The drawing under review shows one solid part. Ordinate dimensions are in mm from its lowest x, y, z. A direction names the side the tool comes from. Coordinates: 2 decimals unless noted, no trailing zeros. Loops run counter-clockwise (first coordinate to the right, second up) from the corner with the lowest first, then second, coordinate; pieces in that order, holes last. Notation, with made-up numbers: (-15, -1) -> (3, -1) arc R13 ccw to (3, 5) -> close; hole circle Ø3 at (64, -33). An arc over 180 degrees is marked (long way). Use a Markdown table: item, result.
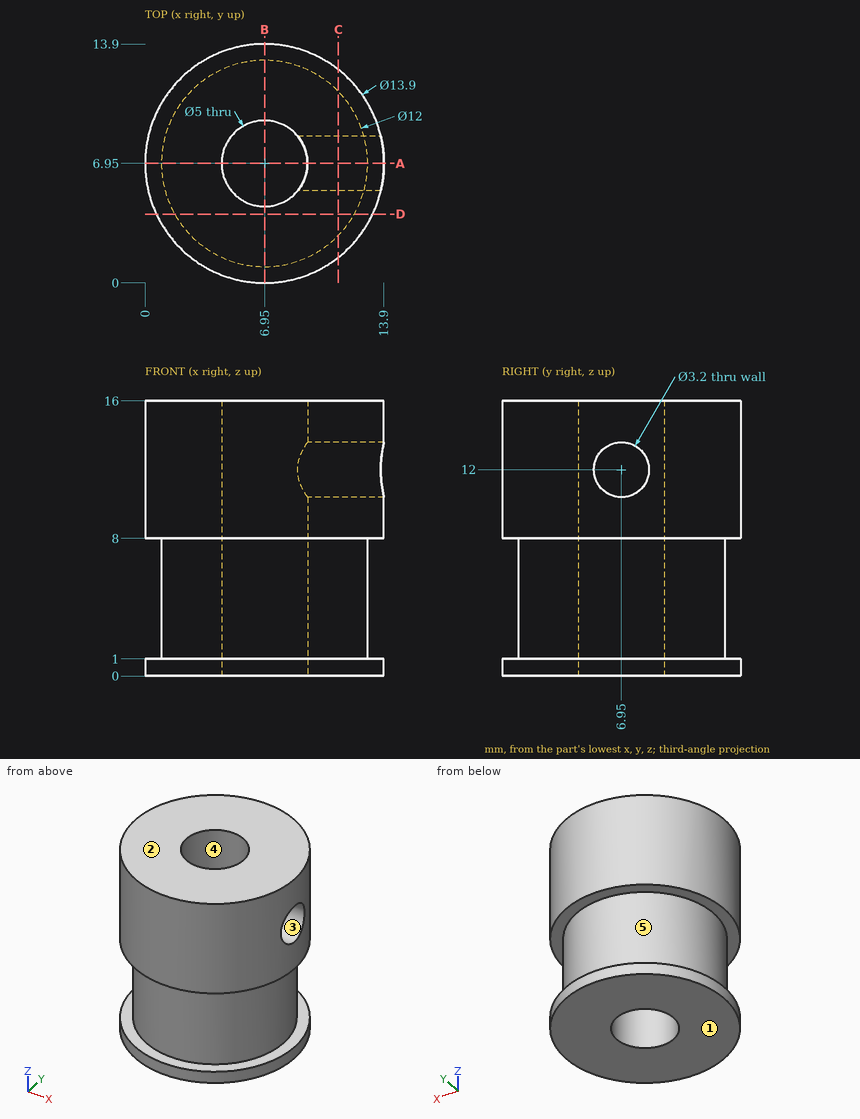
(1) Take a section at B-B on x = 6.95. Write out the cut boundary in (y, z), plus the area to 3 significant figures.
Found:
| item | result |
|---|---|
| outline | (0, 0) -> (4.45, 0) -> (4.45, 16) -> (0, 16) -> (0, 8) -> (0.95, 8) -> (0.95, 1) -> (0, 1) -> close; (9.45, 0) -> (13.9, 0) -> (13.9, 1) -> (12.95, 1) -> (12.95, 8) -> (13.9, 8) -> (13.9, 16) -> (9.45, 16) -> close |
| area | 129 mm^2 |
(2) For line 1 along Y through (x, z) = (6.95, 11.5); line 2 along Z through (x, y) = (11.75, 7); line 3 along Y through (x, z) = (6.95, 5), list the stretches that pass through material, from the lowest coordinate up.
Found:
| item | result |
|---|---|
| line 1 | y = 0 to 4.45, 9.45 to 13.9 |
| line 2 | z = 0 to 10.4, 13.6 to 16 |
| line 3 | y = 0.95 to 4.45, 9.45 to 12.95 |
(3) For pin 1 Ø2 at (y, z) = (5, 6) entering from -X, flat-tipped, find the tip position at first contact; note if it passes through.
Found:
| item | result |
|---|---|
| pin 1 | stops at x = 1.03 |
(4) Take a section at C-C on x = 11.25. Write out the cut boundary in (y, z).
Found:
| item | result |
|---|---|
| outline | (1.49, 0) -> (12.41, 0) -> (12.41, 1) -> (11.13, 1) -> (11.13, 8) -> (12.41, 8) -> (12.41, 16) -> (1.49, 16) -> (1.49, 8) -> (2.77, 8) -> (2.77, 1) -> (1.49, 1) -> close; hole circle Ø3.2 at (6.95, 12) |
(5) Mouldability with a two-part tool opening along Z and no side actions: class the marked faces 1, 2 and 3 as pulls with the +Z half, pulls with the -Z half, needs draft (parallel to the pull), parting line crosses it, or undercut.
Found:
| item | result |
|---|---|
| face 1 | pulls with the -Z half |
| face 2 | pulls with the +Z half |
| face 3 | undercut |
(6) Take a section at D-D on y = 4. Write out the cut boundary in (x, z).
Found:
| item | result |
|---|---|
| outline | (0.66, 0) -> (13.24, 0) -> (13.24, 1) -> (12.17, 1) -> (12.17, 8) -> (13.24, 8) -> (13.24, 16) -> (0.66, 16) -> (0.66, 8) -> (1.73, 8) -> (1.73, 1) -> (0.66, 1) -> close |
(7) Take a section at A-A on y = 6.95. Write out the cut boundary in (x, z), plus the area to 3 significant figures.
Found:
| item | result |
|---|---|
| outline | (0, 0) -> (4.45, 0) -> (4.45, 16) -> (0, 16) -> (0, 8) -> (0.95, 8) -> (0.95, 1) -> (0, 1) -> close; (9.45, 0) -> (13.9, 0) -> (13.9, 1) -> (12.95, 1) -> (12.95, 8) -> (13.9, 8) -> (13.9, 10.4) -> (9.45, 10.4) -> close; (9.45, 13.6) -> (13.9, 13.6) -> (13.9, 16) -> (9.45, 16) -> close |
| area | 115 mm^2 |
(8) For the marked faces 4 and 5, list the 3-axis set-ups (+Z, -Z, +X, -X, +Y, -Y) from which the entire face can be reached by the end or side of a thin tool; tool diameter is ignored.
Found:
| item | result |
|---|---|
| face 4 | +Z, -Z |
| face 5 | none |
